Check sheet for the modelled part. Datum: model origin and axes. Units: mm. Face numbers are marked on the shaded views. A direction names the side the tool comes from. Coordinates: 2 decimals unless noted, no trailing zeros. Loops run counter-clockwise (first coordinate to the right, second up) from the corner with the lowest first, then second, coordinate; pieces in that order, holes last. Notation, with made-up numbers: M -21.75,29 L -14.75,29 A18 cw -14.75,60 Z; hole C 63.5,2 d3. An arc over 180 degrees is marked long. Return JSON: item names as keys, results as strings.
from build123d import *

# Parameters (mm, degrees)
SKETCH_1_W            = 10
SKETCH_1_H            = 83.5
SKETCH_1_R            = 1.6
EXTRUDE_1_DEPTH       = 5
MOVE_START            = -5.1
MOVE_FACE_1_OUTLINE_W = 5
MOVE_FACE_1_OUTLINE_H = 83.5
MOVE_FACE_1_DEPTH     = 0.1
SKETCH_2_W            = 15
SKETCH_2_H            = 5
EXTRUDE_2_DEPTH       = 3
MOVE_START_2          = 5
MOVE_FACE_2_OUTLINE_W = 5
MOVE_FACE_2_OUTLINE_H = 83.5
MOVE_FACE_2_DEPTH     = 0.1
CHAMFER_1_SIZE        = 2
SKETCH_3_W            = 8
SKETCH_3_H            = 10.2
EXTRUDE_3_DEPTH       = 3
EXTRUDE_4_DEPTH       = 73.5


# Read off the part's stored shape, not the designer's step: 面の移動1, 面の移動2
with BuildPart() as part:
    # ｽｹｯﾁ1 → ﾎﾞｽ - 押し出し1 (new body)
    with BuildSketch(Plane.ZY.offset(7.5)):
        with Locations((0, -68.25)):
            Rectangle(SKETCH_1_W, SKETCH_1_H)
        with Locations((0, -74)):
            Circle(SKETCH_1_R, mode=Mode.SUBTRACT)
        with Locations((0, -34)):
            Circle(SKETCH_1_R, mode=Mode.SUBTRACT)
    extrude(amount=EXTRUDE_1_DEPTH)

    # Move Face 1 outline → Move Face 1 (add)
    with BuildSketch(Plane.XY.offset(MOVE_START)):
        with Locations((-10, -68.25)):
            Rectangle(MOVE_FACE_1_OUTLINE_W, MOVE_FACE_1_OUTLINE_H)
    extrude(amount=MOVE_FACE_1_DEPTH)

    # ｽｹｯﾁ2 → ﾎﾞｽ - 押し出し2 (add)
    with BuildSketch(Plane(origin=(0, 0, -5.1), x_dir=(-1, 0, 0), z_dir=(0, 0, -1))):
        with Locations((5, -107.5)):
            Rectangle(SKETCH_2_W, SKETCH_2_H)
        with Locations((5, -29)):
            Rectangle(SKETCH_2_W, SKETCH_2_H)
        with Locations((5, -68.25)):
            Rectangle(SKETCH_2_W, SKETCH_2_H)
    extrude_2 = extrude(amount=EXTRUDE_2_DEPTH)

    # Move Face 2 outline → Move Face 2 (add)
    with BuildSketch(Plane.XY.offset(MOVE_START_2)):
        with Locations((-10, -68.25)):
            Rectangle(MOVE_FACE_2_OUTLINE_W, MOVE_FACE_2_OUTLINE_H)
    extrude(amount=MOVE_FACE_2_DEPTH)

    # ﾐﾗｰ2: ﾎﾞｽ - 押し出し2 across plane
    add(extrude_2.mirror(Plane.XY))

    # 面取り1
    chamfer_1_edges = [part.edges().sort_by_distance(p)[0] for p in [
        (2.5, -107.5, -5.1),
        (2.5, -29, -5.1),
        (2.5, -68.25, -5.1),
        (2.5, -107.5, 5.1),
        (2.5, -29, 5.1),
        (2.5, -68.25, 5.1),
    ]]
    chamfer(chamfer_1_edges, length=CHAMFER_1_SIZE)

    # ｽｹｯﾁ3 → ﾎﾞｽ - 押し出し3 (add)
    with BuildSketch(Plane.XZ.offset(110)):
        Polygon((-7.5, -5.1), (-7.5, 5.1), (0.5, 5.1), (2.5, 7.1), (2.5, 8.1), (-12.5, 8.1), (-12.5, -8.1), (2.5, -8.1), (2.5, -7.1), (0.5, -5.1), align=None)
        with Locations((-3.5, 0)):
            Rectangle(SKETCH_3_W, SKETCH_3_H)
    extrude(amount=EXTRUDE_3_DEPTH)

    # ｽｹｯﾁ4 → ﾎﾞｽ - 押し出し4 (add)
    with BuildSketch(Plane.XZ.offset(31.5)):
        Polygon((-7.5, 5.1), (0.5, 5.1), (2.5, 7.1), (2.5, 8.1), (-12.5, 8.1), (-12.5, 5.1), align=None)
        Polygon((2.5, -8.1), (2.5, -7.1), (0.5, -5.1), (-7.5, -5.1), (-12.5, -5.1), (-12.5, -8.1), align=None)
    extrude(amount=EXTRUDE_4_DEPTH)


solid = part.part
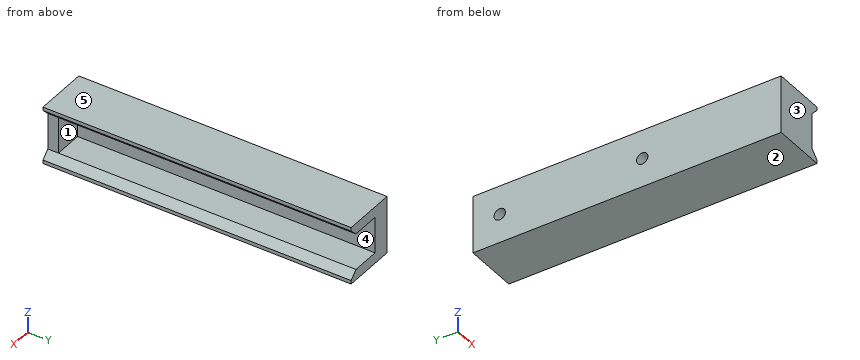
1) Set-up check for the marked faces 4 and 5: record each of +Z, -Z, +X, -X, +Y, -Y from which the full face is reachable in a straight line by a thin tool's end or side.
Answers:
{"face 4": "+X, +Y", "face 5": "+Z, +X, -X, +Y, -Y"}
2) Section check B-B on z = 0. Record the cut outline in (x, y).
Answers:
{"outline": "M -12.5,-113 L 0.5,-113 L 0.5,-110 L -7.5,-110 L -7.5,-75.6 L -12.5,-75.6 Z; M -12.5,-72.4 L -7.5,-72.4 L -7.5,-35.6 L -12.5,-35.6 Z; M -12.5,-32.4 L -7.5,-32.4 L -7.5,-26.5 L -12.5,-26.5 Z"}
3) Go/stop test with flat-tipped pins: pin 1 Ø3.5 at (y, z) = (-111.5, 0) entering from +X; pin 2 Ø3 at (y, z) = (-34, 0) entering from -X; pin 3 Ø6.5 at (x, z) = (-4, 1.5) entering from +Y; pin 4 Ø4 at (y, z) = (-52, -3) entering from +X. Record where each tip stops, or that it passes through.
Answers:
{"pin 1": "x = 0.5", "pin 2": "through", "pin 3": "y = -110", "pin 4": "x = -7.5"}
4) Section check D-D on y = -78.5. Record the cut outline in (x, z).
Answers:
{"outline": "M -12.5,-8.1 L 2.5,-8.1 L 2.5,-7.1 L 0.5,-5.1 L -7.5,-5.1 L -7.5,5.1 L 0.5,5.1 L 2.5,7.1 L 2.5,8.1 L -12.5,8.1 Z"}
5) Section check C-C on y = -34. Record the cut outline in (x, z), then the cut area to 3 significant figures.
Answers:
{"outline": "M -12.5,-8.1 L 2.5,-8.1 L 2.5,-7.1 L 0.5,-5.1 L -7.5,-5.1 L -7.5,-1.6 L -12.5,-1.6 Z; M -12.5,1.6 L -7.5,1.6 L -7.5,5.1 L 0.5,5.1 L 2.5,7.1 L 2.5,8.1 L -12.5,8.1 Z", "area": "121 mm²"}
6) Section check A-A on x = 1.5. Record the cut outline in (y, z).
Answers:
{"outline": "M -113,-8.1 L -26.5,-8.1 L -26.5,-6.1 L -113,-6.1 Z; M -113,6.1 L -26.5,6.1 L -26.5,8.1 L -113,8.1 Z"}
7) Draft check along Z on the marked faces 1, 2 and 3. Enter one of: +Z half, -Z half, draft (parallel to the pull), parting line (faces both ways), or undercut.
Answers:
{"face 1": "undercut", "face 2": "-Z half", "face 3": "draft"}
8) Scan lines: line 1 along Y through (x, z) = (-11.1, 0); line 2 along Z through (x, y) = (-10.1, -74); line 3 along Z through (x, y) = (-3.5, -83). Record each from-to range of solid material in increasing order. Write a range as [from, to].
Answers:
{"line 1": "[-113, -75.6], [-72.4, -35.6], [-32.4, -26.5]", "line 2": "[-8.1, -1.6], [1.6, 8.1]", "line 3": "[-8.1, -5.1], [5.1, 8.1]"}
